Check sheet for the modelled part. Datum: model origin and axes. Units: mm. A direction names the side the tool comes from. Give positions to 0.01 mm unless a question says otherwise; leave off trailing zeros. Write each loop counter-clockwise with the first axis right and the second up, starting at its lowest first coordinate (ties: lowest second). Pieces come first, ordered by that corner, then holes.
Solid Edge part; units mm, degrees
sketch "Sketch1" plane through (0, 0, 0) normal (0, -1, 0) x (1, 0, 0)
  line L0 (67.5, -10) -> (67.5, -20)
  line L1 (67.5, -20) -> (27.5, -20)
  line L2 (27.5, -20) -> (27.5, -10)
  line L3 (27.5, -10) -> (3, -10)
  line L4 (3, -10) -> (0, -10)
  line L5 (0, -10) -> (-3, -10)
  line L6 (-3, -10) -> (-27.5, -10)
  line L7 (-27.5, -10) -> (-27.5, -20)
  line L8 (-27.5, -20) -> (-37.5, -20)
  line L9 (-37.5, -20) -> (-52.5, -20)
  line L10 (-52.5, -20) -> (-67.5, -20)
  line L11 (-67.5, -20) -> (-67.5, -10)
  line L12 (-67.5, -10) -> (-37.5, -10)
  line L13 (-37.5, -10) -> (-37.5, 0)
  line L14 (-37.5, 0) -> (-27.5, 0)
  line L15 (-27.5, 0) -> (-15.8209, 0)
  line L16 (-15.8209, 0) -> (0, 0)
  line L17 (0, 0) -> (3, 0)
  line L18 (3, 0) -> (27.5, 0)
  line L19 (27.5, 0) -> (37.5, 0)
  line L20 (37.5, 0) -> (37.5, -10)
  line L21 (37.5, -10) -> (52.5, -10)
  line L22 (52.5, -10) -> (67.5, -10)
extrude "Protrusion1" add sketch "Sketch1" against normal blind 90
sketch "Sketch2" plane through (0, 0, 0) normal (1, 0, 0) x (0, 1, 0)
  line L0 (90, 45) -> (90, 0)
  line L1 (90, 0) -> (50, 0)
  line L2 (50, 0) -> (50, 45)
  arc A0 (50, 45) -> (90, 45) centre (70, 45) cw
extrude "ExtrudedProtrusion_5" add sketch "Sketch2" along normal mid plane 75
sketch "Sketch3" plane through (0, 0, 0) normal (1, 0, 0) x (0, 1, 0)
  circle A0 centre (70, 45) radius 10
extrude "ExtrudedCutout_1" cut sketch "Sketch3" along normal mid plane 75
sketch "Sketch4" plane through (0, 0, 0) normal (1, 0, 0) x (0, 1, 0)
  line L0 (0, 0) -> (55.4585, 58.7312)
  line L1 (50, 45) -> (50, 0)
  line L2 (50, 0) -> (0, 0)
  arc A0 (50, 45) -> (55.4585, 58.7312) centre (70, 45) cw
extrude "ExtrudedProtrusion_6" add sketch "Sketch4" along normal mid plane 6
sketch "Sketch5" plane through (0, 0, -10) normal (0, -1, 0) x (1, 0, 0)
  line L0 (67.5, 0) -> (37.5, 10)
  line L1 (37.5, 10) -> (37.5, 0)
  line L2 (37.5, 0) -> (67.5, 0)
extrude "ExtrudedProtrusion_7" add sketch "Sketch5" against normal blind 43
sketch "Sketch6" plane through (0, 0, -10) normal (0, -1, 0) x (1, 0, 0)
  line L0 (67.5, 0) -> (37.5, 10)
  line L1 (37.5, 10) -> (37.5, 0)
  line L2 (37.5, 0) -> (67.5, 0)
extrude "ExtrudedCutout_2" cut sketch "Sketch6" against normal blind 37
sketch "Sketch7" plane through (0, 0, -10) normal (0, -1, 0) x (1, 0, 0)
  line L0 (-67.5, 0) -> (-37.5, 10)
  line L1 (-37.5, 10) -> (-37.5, 0)
  line L2 (-37.5, 0) -> (-67.5, 0)
extrude "ExtrudedProtrusion_8" add sketch "Sketch7" against normal blind 43
sketch "Sketch8" plane through (0, 0, -10) normal (0, -1, 0) x (1, 0, 0)
  line L0 (-67.5, 0) -> (-37.5, 10)
  line L1 (-37.5, 10) -> (-37.5, 0)
  line L2 (-37.5, 0) -> (-67.5, 0)
extrude "ExtrudedCutout_3" cut sketch "Sketch8" against normal blind 37
sketch "Sketch9" plane through (52.5, 18.5, -10) normal (0, 0, 1) x (0, 1, 0)
  circle A0 centre (1.5, 0) radius 6
extrude "ExtrudedCutout_4" cut sketch "Sketch9" against normal blind 10
sketch "Sketch10" plane through (52.5, 18.5, -10) normal (0, 0, 1) x (0, 1, 0)
  circle A0 centre (51.5, 0) radius 6
extrude "ExtrudedCutout_5" cut sketch "Sketch10" against normal blind 10
sketch "Sketch11" plane through (52.5, 18.5, -10) normal (0, 0, 1) x (0, 1, 0)
  circle A0 centre (51.5, 105) radius 6
extrude "ExtrudedCutout_6" cut sketch "Sketch11" against normal blind 10
sketch "Sketch12" plane through (52.5, 18.5, -10) normal (0, 0, 1) x (0, 1, 0)
  circle A0 centre (1.5, 105) radius 6
extrude "ExtrudedCutout_8" cut sketch "Sketch12" against normal blind 10
1) Gauge pin test, flat ends, axial feed: pin 1 (10 mm diameter, centred on x = -47.5, z = -1.5, fed in from -Y); pin 2 (5 mm diameter, centred on y = 18, z = -3, fed in from +X); pin 3 (16.5 mm diameter, centred on x = -4, y = 52.5, fed in from -Z). Record the tip position at first contact, or that the pin passes through.
2) Sectioned sample at C-C on x = 10. Record the boundary of the cut face in (y, z), then the cut area to 3 significant figures.
3) Access from +Z, -Z, +X, -X, +Y, -Y to the whole of each face (thin tool, end or side, straight path). Record for faces 5 (the flat face through (37.5, 18, -5)), 6 (the flat face through (-37.5, 66, 19)), 7 (the flat face through (27.5, 44, -15)).
4) Sectioned sample at B-B on y = 70. Record the boundary of the cut face in (x, z).
5) Scan lines: L1, parallel to X at y = 20, z = -13.25; L2, parallel to Y at x = -52.5, z = -15.5; L3, parallel to X at y = 51.5, z = 24.5. Record each from-to range of solid material in increasing order.
6) Draft check along Z on faces 1 (the flat face through (52, 61, -10)), 2 (the cylindrical face through (-1, 62, 51)), 3 (the flat face through (-37.5, 18, -5)), 4 (the flat face through (48, 44, -20)). Enter one of: +Z half, -Z half, draft (parallel to the pull), parting line (faces both ways), or undercut.
7) Sectioned sample at D-D on z = 48.5. Record the boundary of the cut face in (x, y).
8) Sectioned sample at A-A on x = 52.5. Record the boundary of the cut face in (y, z), then the cut area to 3 significant figures.
Answers below:
1. pin 1: stops at y = 37
1. pin 2: stops at x = 37.5
1. pin 3: stops at z = -10
2. outline: (0, -10) - (90, -10) - (90, 45) arc R20 ccw to (50, 45) - (50, 0) - (0, 0) - close; hole circle Ø20 at (70, 45)
2. area: 3,010 mm2
3. face 5: +Z, +X, -Y
3. face 6: +Z, -X, +Y
3. face 7: -Z, +Y, -Y
4. outline: (-67.5, -20) - (-58.5, -20) - (-58.5, -10) - (-67.5, -10) - close; (-46.5, -20) - (-27.5, -20) - (-27.5, -10) - (27.5, -10) - (27.5, -20) - (46.5, -20) - (46.5, -10) - (37.5, -10) - (37.5, 35) - (-37.5, 35) - (-37.5, -10) - (-46.5, -10) - close; (-37.5, 55) - (37.5, 55) - (37.5, 65) - (-37.5, 65) - close; (58.5, -20) - (67.5, -20) - (67.5, -10) - (58.5, -10) - close
5. L1: x = -67.5 to -58.5, -46.5 to -27.5, 27.5 to 46.5, 58.5 to 67.5
5. L2: y = 0 to 14, 26 to 64, 76 to 90
5. L3: x = -37.5 to 37.5
6. face 1: +Z half
6. face 2: undercut
6. face 3: draft
6. face 4: -Z half
7. outline: (-37.5, 50.31) - (-3, 50.31) - (-3, 45.8) - (3, 45.8) - (3, 50.31) - (37.5, 50.31) - (37.5, 60.63) - (-37.5, 60.63) - close; (-37.5, 79.37) - (37.5, 79.37) - (37.5, 89.69) - (-37.5, 89.69) - close
8. outline: (0, -20) - (14, -20) - (14, -10) - (0, -10) - close; (26, -20) - (64, -20) - (64, -10) - (43, -10) - (43, -5) - (37, -5) - (37, -10) - (26, -10) - close; (76, -20) - (90, -20) - (90, -10) - (76, -10) - close
8. area: 690 mm2
